from build123d import *

# Parameters (mm, degrees)
SKETCH_1_R          = 30
SKETCH_1_R_2        = 3.05
SKETCH_1_R_3        = 6
EXTRUDE_1_DEPTH     = 20
SKETCH_2_W          = 22
SKETCH_2_H          = 22
CUT_EXTRUDE_1_DEPTH = 10
SKETCH_3_R          = 5.95
CUT_EXTRUDE_6_DEPTH = 10


with BuildPart() as part:
    # Эскиз1 → Бобышка-Вытянуть1 (new body)
    with BuildSketch(Plane.XY):
        Circle(SKETCH_1_R)
        with Locations((0, 24)):
            Circle(SKETCH_1_R_2, mode=Mode.SUBTRACT)
        with Locations((20.784609691, 12)):
            Circle(SKETCH_1_R_2, mode=Mode.SUBTRACT)
        with Locations((20.784609691, -12)):
            Circle(SKETCH_1_R_2, mode=Mode.SUBTRACT)
        with Locations((0, -24)):
            Circle(SKETCH_1_R_2, mode=Mode.SUBTRACT)
        with Locations((-20.784609691, -12)):
            Circle(SKETCH_1_R_2, mode=Mode.SUBTRACT)
        with Locations((-20.784609691, 12)):
            Circle(SKETCH_1_R_2, mode=Mode.SUBTRACT)
        Circle(SKETCH_1_R_3, mode=Mode.SUBTRACT)
    extrude(amount=EXTRUDE_1_DEPTH)

    # Эскиз2 → Вырез-Вытянуть1 (cut)
    with BuildSketch(Plane.XY.offset(20)):
        Rectangle(SKETCH_2_W, SKETCH_2_H)
    extrude(amount=-CUT_EXTRUDE_1_DEPTH, mode=Mode.SUBTRACT)

    # Эскиз3 → Вырез-Вытянуть6 (cut)
    with BuildSketch(Plane(origin=(0, 0, 0), x_dir=(-1, 0, 0), z_dir=(0, 0, -1))):
        with Locations((0, 24)):
            Circle(SKETCH_3_R)
        with Locations((20.784609691, 12)):
            Circle(SKETCH_3_R)
        with Locations((20.784609691, -12)):
            Circle(SKETCH_3_R)
        with Locations((0, -24)):
            Circle(SKETCH_3_R)
        with Locations((-20.784609691, -12)):
            Circle(SKETCH_3_R)
        with Locations((-20.784609691, 12)):
            Circle(SKETCH_3_R)
    extrude(amount=-CUT_EXTRUDE_6_DEPTH, mode=Mode.SUBTRACT)


solid = part.part
CAD build for the part. Positions are in the model's coordinates, mm. A direction names the side the tool comes from. Round coordinates to 2 decimals unless told otherwise and drop trailing zeros. Write each loop counter-clockwise with the first axis right and the second up, starting at its lowest first coordinate (ties: lowest second). Pieces come first, ordered by that corner, then holes.
(1) 3-axis set-ups, long thin cutter, end or side, ignore diameter. For faces 4 (the face through (-6, 0, 5)), 5 (the face through (-5, -5, 10)), 6 (the face through (-3, -27, 10)): which of +Z, -Z, +X, -X, +Y, -Y reach the whole face in a straight line?
(2) Probe line 1 along Y through (x, z) = (19.5, 14.25); line 2 along X through (y, z) = (-1.5, 15.25); line 3 along X through (y, z) = (-12.5, 6.75). List the from-to ranges inside material, lowest first.
(3) Slice it at B-B, the plane y = 12. Write the cut outline in (x, z), and give its area (3 significant figures).
(4) Mould opens along X. For faces 1 (the face through (-0.4, -6.2, 0)), 2 (the face through (-29.97, 1.32, 9.86)), 3 (the face through (24, -11, 10)) say: pulls with the +X half, pulls with the -X half, needs draft (parallel to the pull), parting line crosses it, or undercut.
(5) Slice it at D-D, the plane y = 0. Write the cut outline in (x, z), and give its area (3 significant figures).
(6) Slice it at A-A, the plane z = 7.5. Write the cut outline in (x, y).
(7) Drop flat-ended pins along their axis: P1, Ø10, axis at x = 5.5, z = 2.5, coming from the +Y side; P2, Ø10, axis at x = -12, z = 7.5, coming from the +Y side; P3, Ø3.5, axis at x = -22, y = 14, coming from the -Z side; P4, Ø5, axis at x = -21, y = -12, coming from the +Z side. Give the stop position or say it passes through.
(8) Slice it at C-C, the plane x = 0. Write the cut outline in (y, z).
From the geometry:
1. face 4: +Z, -Z
1. face 5: +Z
1. face 6: -Z
2. line 1: y = -22.8 to -14.77, -9.23 to 9.23, 14.77 to 22.8
2. line 2: x = -29.96 to -11, 11 to 29.96
2. line 3: x = -27.27 to -26.71, -14.86 to 14.86, 26.71 to 27.27
3. outline: (-27.5, 0) - (-26.73, 0) - (-26.73, 10) - (-23.83, 10) - (-23.83, 20) - (-27.5, 20) - close; (-17.73, 10) - (-14.83, 10) - (-14.83, 0) - (14.83, 0) - (14.83, 10) - (17.73, 10) - (17.73, 20) - (-17.73, 20) - close; (23.83, 10) - (26.73, 10) - (26.73, 0) - (27.5, 0) - (27.5, 20) - (23.83, 20) - close
3. area: 740 mm2
4. face 1: needs draft
4. face 2: parting line crosses it
4. face 3: undercut
5. outline: (-30, 0) - (-6, 0) - (-6, 10) - (-11, 10) - (-11, 20) - (-30, 20) - close; (6, 0) - (30, 0) - (30, 20) - (11, 20) - (11, 10) - (6, 10) - close
5. area: 860 mm2
6. outline: circle Ø60 at (0, 0); hole circle Ø11.9 at (-20.78, -12); hole circle Ø11.9 at (-20.78, 12); hole circle Ø12 at (0, 0); hole circle Ø11.9 at (0, -24); hole circle Ø11.9 at (0, 24); hole circle Ø11.9 at (20.78, -12); hole circle Ø11.9 at (20.78, 12)
7. P1: stops at y = 30
7. P2: stops at y = 29.17
7. P3: stops at z = 10
7. P4: passes through
8. outline: (-30, 0) - (-29.95, 0) - (-29.95, 10) - (-27.05, 10) - (-27.05, 20) - (-30, 20) - close; (-20.95, 10) - (-18.05, 10) - (-18.05, 0) - (-6, 0) - (-6, 10) - (-11, 10) - (-11, 20) - (-20.95, 20) - close; (6, 0) - (18.05, 0) - (18.05, 10) - (20.95, 10) - (20.95, 20) - (11, 20) - (11, 10) - (6, 10) - close; (27.05, 10) - (29.95, 10) - (29.95, 0) - (30, 0) - (30, 20) - (27.05, 20) - close
